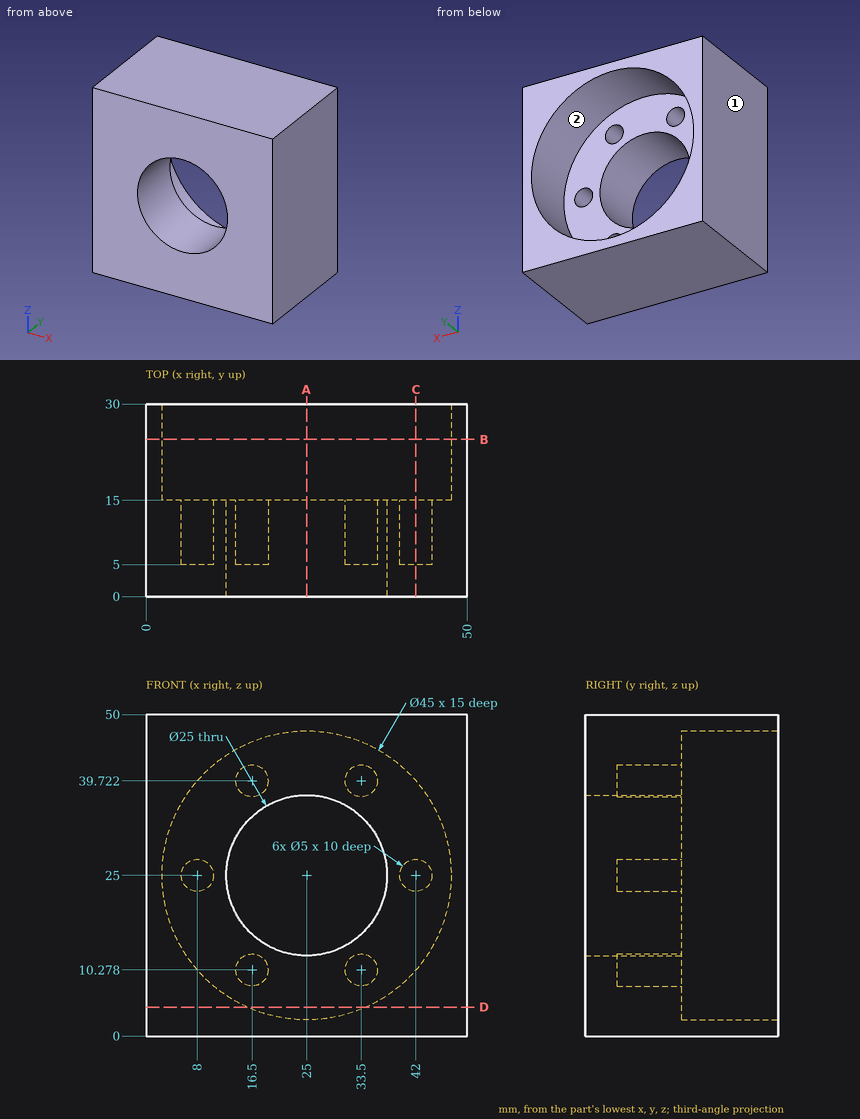
Study the drawing (mm; zero at the part's minimum x, y, z) and answer. A direction names the side the tool comes from. Give positions to 0.01 mm unless a question says otherwise; leave off trailing zeros. Write each loop counter-clockwise with the first axis right and the second up, starting at its lowest first coordinate (ties: lowest second). Pieces come first, ordered by that corner, then holes. Notation, with made-up numbers: (26, 0.5) -> (39, 0.5) arc R27 ccw to (39, 37.5) -> close; hole circle Ø5 at (32, 73.5). An arc over 180 degrees is marked (long way). Write item = value, one per line.
Q1. Consider line 1 along X through (y, z) = (12.25, 25); line 2 along Z through (x, y) = (25, 4.75); line 3 along Z through (x, y) = (33.5, 10.5) (1 decimal). Determine where each line is inside the solid, lowest interval first.
Computed values:
line_1 = 0 to 5.5, 10.5 to 12.5, 37.5 to 39.5, 44.5 to 50
line_2 = 0 to 12.5, 37.5 to 50
line_3 = 0 to 7.8, 12.8 to 15.8, 34.2 to 37.2, 42.2 to 50
Q2. Section A-A on x = 25 is taken. Determine the outline of the cut face in (y, z).
Computed values:
outline = (0, 0) -> (30, 0) -> (30, 2.5) -> (15, 2.5) -> (15, 12.5) -> (0, 12.5) -> close; (0, 37.5) -> (15, 37.5) -> (15, 47.5) -> (30, 47.5) -> (30, 50) -> (0, 50) -> close
Q3. A tool of negligible diameter and unlimited length cuts with its end or side. For the marked faces 1 and 2, from which of +Z, -Z, +X, -X, +Y, -Y can it reach the whole face along a straight path? Write none if from no direction.
Computed values:
face_1 = +Z, -Z, -X, +Y, -Y
face_2 = +Y
Q4. Section C-C on x = 42 is taken. Determine the outline of the cut face in (y, z), and give its area (3 significant figures).
Computed values:
outline = (0, 0) -> (30, 0) -> (30, 10.26) -> (15, 10.26) -> (15, 22.5) -> (5, 22.5) -> (5, 27.5) -> (15, 27.5) -> (15, 39.74) -> (30, 39.74) -> (30, 50) -> (0, 50) -> close
area = 1,010 mm^2
Q5. Section B-B on y = 24.5 is taken. Determine the outline of the cut face in (x, z).
Computed values:
outline = (0, 0) -> (50, 0) -> (50, 50) -> (0, 50) -> close; hole circle Ø45 at (25, 25)
Q6. Section D-D on z = 4.5 is taken. Determine the outline of the cut face in (x, y).
Computed values:
outline = (0, 0) -> (50, 0) -> (50, 30) -> (34.27, 30) -> (34.27, 15) -> (15.73, 15) -> (15.73, 30) -> (0, 30) -> close
Q7. Flat-ended cylindrical pins translate along their axes: pin 1 Ø3 at (x, z) = (16.5, 10.28) entering from +Y; pin 2 Ø4 at (x, z) = (32.5, 10.5) entering from +Y; pin 3 Ø20 at (x, z) = (25, 25) entering from -Y. Find the tip coordinate at first contact, or state that the pin passes through.
Computed values:
pin_1 = 5
pin_2 = 15
pin_3 = through
